Part print with two shaded views. Sizes in mm from the minimum x, y, z corner. A direction names the side the tool comes from. Coordinates: 2 decimals unless noted, no trailing zeros. Loops run counter-clockwise (first coordinate to the right, second up) from the corner with the lowest first, then second, coordinate; pieces in that order, holes last. Notation, with made-up numbers: (36.25, -6.75) -> (58.25, -6.75) arc R16 ccw to (58.25, 2.25) -> close; hole circle Ø8 at (-31, 89). An arc over 180 degrees is marked (long way). Write each question's results on one line, items separated by ' | '.
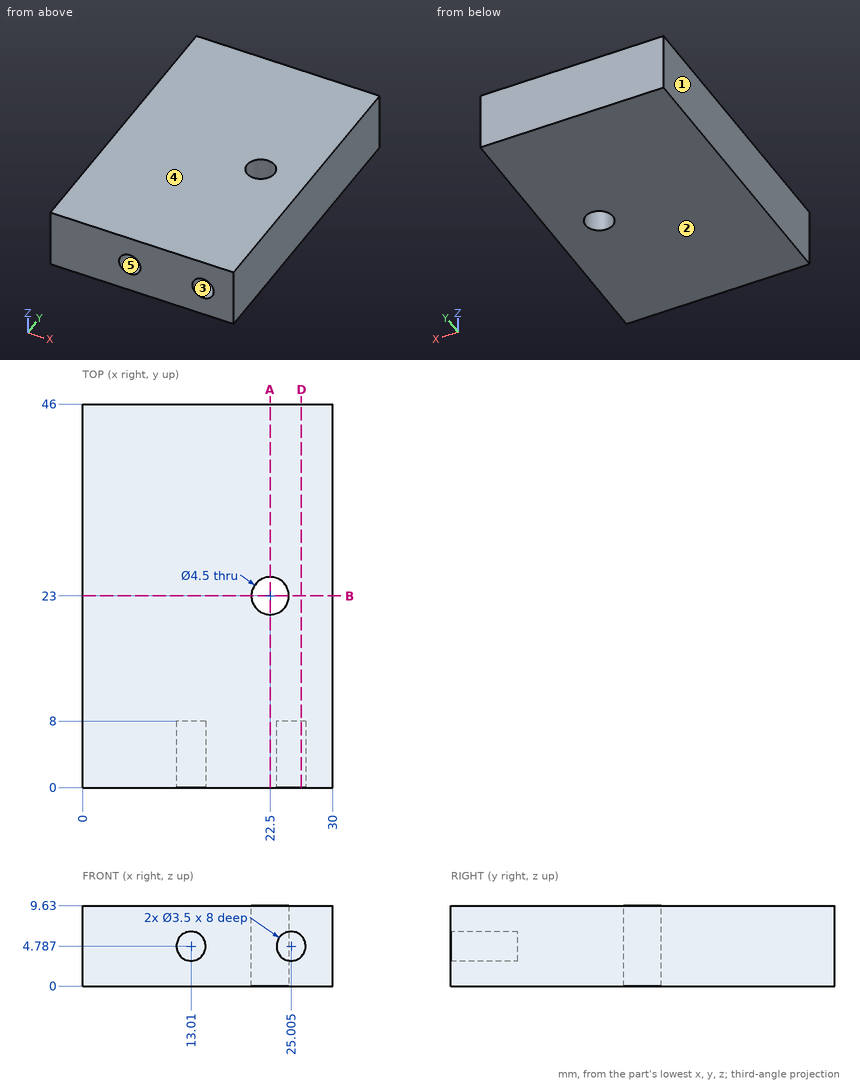
Q1. Cut at D-D on x = 26.25. Write the cut outline in (y, z).
Results are:
outline: (0, 0) -> (46, 0) -> (46, 9.63) -> (0, 9.63) -> (0, 6.02) -> (8, 6.02) -> (8, 3.56) -> (0, 3.56) -> close
Q2. Drop a flat-ended pin along its axis: pin 1 (1.8 mm diameter, centred on x = 12.5, z = 5, fed in from -Y). Give the stop position or say it passes through.
Results are:
pin 1: y = 8
Q3. Wall check: L1, parallel to Y at x = 22.5, z = 3.25; L2, parallel to X at y = 3.5, z = 4; L3, parallel to Y at x = 23.75, z = 4. Give the ranges that are in metal, low to high. Write a range as from..to.
Results are:
L1: 0..20.75, 25.25..46 | L2: 0..11.45, 14.57..23.44, 26.57..30 | L3: 8..21.13, 24.87..46
Q4. Pull direction X, two halves, no side cores. Call the marked faces 1, 2 and 3: +X half, -X half, draft (parallel to the pull), parting line (faces both ways), or undercut.
Results are:
face 1: -X half | face 2: draft | face 3: undercut
Q5. Which spindle directions (+Z, -Z, +X, -X, +Y, -Y) get a long thin tool onto all of the face, cutting with end or side? Do the marked faces 4 and 5. Say none if no direction does.
Results are:
face 4: +Z, +X, -X, +Y, -Y | face 5: -Y
Q6. Cut at A-A on x = 22.5. Write the cut outline in (y, z), and give its area (3 significant figures).
Results are:
outline: (0, 0) -> (20.75, 0) -> (20.75, 9.63) -> (0, 9.63) -> close; (25.25, 0) -> (46, 0) -> (46, 9.63) -> (25.25, 9.63) -> close | area: 400 mm^2
Q7. Cut at B-B on y = 23. Write the cut outline in (x, z).
Results are:
outline: (0, 0) -> (20.25, 0) -> (20.25, 9.63) -> (0, 9.63) -> close; (24.75, 0) -> (30, 0) -> (30, 9.63) -> (24.75, 9.63) -> close
